from build123d import *

# Parameters (mm, degrees)
F0_W     = 35
F0_H     = 350
F0_R     = 5
F1_DEPTH = 15
F2_W     = 15
F2_H     = 350
F3_DEPTH = 109
F5_DEPTH = 15
F7_DEPTH = 5


with BuildPart() as f1:
    # F0 (on Top) → F1 (new body)
    with BuildSketch(Plane.XY):
        with Locations((-57.72887, 129.090141)):
            Rectangle(F0_W, F0_H)
        with Locations((-50.22887, -15.909859)):
            Circle(F0_R, mode=Mode.SUBTRACT)
        with Locations((-50.22887, 129.090141)):
            Circle(F0_R, mode=Mode.SUBTRACT)
        with Locations((-50.22887, 274.090141)):
            Circle(F0_R, mode=Mode.SUBTRACT)
    extrude(amount=F1_DEPTH)

    # F2 (on face) → F3 (join)
    with BuildSketch(Plane.XY.offset(15)):
        with Locations((-67.72887, 129.090141)):
            Rectangle(F2_W, F2_H)
    extrude(amount=F3_DEPTH)

    # F4 (on face) → F5 (join)
    with BuildSketch(Plane.YZ.offset(-60.22887)):
        Polygon((254.726105, 303.215003), (-45.909859, 124), (304.090141, 124), (304.090141, 332.641874), align=None)
    extrude(amount=-F5_DEPTH)

    # F6 (on face) → F7 (cut)
    with BuildSketch(Plane(origin=(-75.22887, 0, 0), x_dir=(0, -1, 0), z_dir=(-1, 0, 0))):
        Polygon((36.23861, 117.541139), (39.054846, 122.265419), (-304.090141, 326.820885), (-304.090141, 320.417792), align=None)
    extrude(amount=-F7_DEPTH, mode=Mode.SUBTRACT)


solid = f1.part
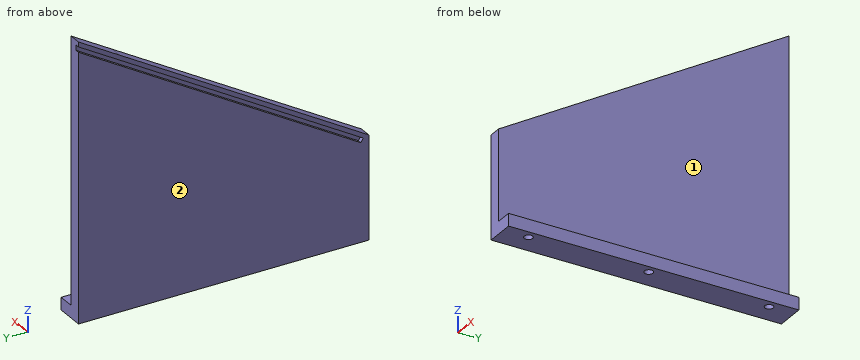
For this review, take the finished solid that the model builds, in its own axes (mm). Face numbers are marked on the shaded views. A direction names the side the tool comes from. Round coordinates to 2 decimals unless told otherwise and drop trailing zeros. Write each loop counter-clockwise with the first axis right and the second up, starting at its lowest first coordinate (ties: lowest second). Pieces come first, ordered by that corner, then holes. Notation, with made-up numbers: (9, 63.5) - (55, 63.5) arc R17 cw to (55, 75.5) - close; hole circle Ø4 at (-15.75, -27). An arc over 180 degrees is marked (long way). Use a Markdown table: item, result.
Q1. Wall thickness on line 1 along Z through (x, y) = (-52, 183.5); line 2 along X through (y, z) = (-18, 119); line 3 along Y through (x, z) = (-72, 221.5): over which ranges is each line inside the solid? List them lowest first.
Derived:
| item | result |
|---|---|
| line 1 | z = 0 to 15 |
| line 2 | x = -75.23 to -60.23 |
| line 3 | y = 117.65 to 127.41, 138.15 to 304.09 |
Q2. Machinability: for the marked faces 1 and 2, which of the approach directions +Z, -Z, +X, -X, +Y, -Y give a long, thin tool a straight path to every point of the face, cutting with its end or side? Answer none if there is none.
Derived:
| item | result |
|---|---|
| face 1 | +Z, +X, +Y, -Y |
| face 2 | +Z, -Z, -X, +Y, -Y |
Q3. Clearance check with flat-ended pins moving along their axes: pin 1 (2 mm diameter, centred on x = -51.5, y = 44.5, fed in from +Z); pin 2 (1 mm diameter, centred on x = -61.5, y = 85, fed in from -Z); pin 3 (2 mm diameter, centred on x = -59.5, y = 182.5, fed in from +Z); pin 4 (8 mm diameter, centred on x = -50.23, y = 274.09, fed in from +Z). State where each tip first meets the part, or that it passes through.
Derived:
| item | result |
|---|---|
| pin 1 | stops at z = 15 |
| pin 2 | stops at z = 0 |
| pin 3 | stops at z = 260.57 |
| pin 4 | passes through |
Q4. We need section B-B (z = 219). Give the boundary of the cut face in (x, y), plus the area to 3 significant figures.
Derived:
| item | result |
|---|---|
| outline | (-75.23, 113.45) - (-60.23, 113.45) - (-60.23, 304.09) - (-75.23, 304.09) - (-75.23, 133.96) - (-70.23, 133.96) - (-70.23, 123.22) - (-75.23, 123.22) - close |
| area | 2,810 mm2 |
Q5. We need section C-C (x = -65.5). Give the boundary of the cut face in (y, z) (3 decimals), plus the area to 3 significant figures.
Derived:
| item | result |
|---|---|
| outline | (-45.91, 0) - (304.09, 0) - (304.09, 332.642) - (-45.91, 124) - close |
| area | 79,900 mm2 |
Q6. We need section D-D (y = 238.5). Give the boundary of the cut face in (x, z), plus the area to 3 significant figures.
Derived:
| item | result |
|---|---|
| outline | (-75.23, 0) - (-40.23, 0) - (-40.23, 15) - (-60.23, 15) - (-60.23, 293.54) - (-75.23, 293.54) - (-75.23, 287.72) - (-70.23, 287.72) - (-70.23, 281.32) - (-75.23, 281.32) - close |
| area | 4,670 mm2 |
Q7. We need section A-A (y = 48.5). Give the boundary of the cut face in (x, z), plus the area to 3 significant figures.
Derived:
| item | result |
|---|---|
| outline | (-75.23, 0) - (-40.23, 0) - (-40.23, 15) - (-60.23, 15) - (-60.23, 180.28) - (-75.23, 180.28) - (-75.23, 174.46) - (-70.23, 174.46) - (-70.23, 168.06) - (-75.23, 168.06) - close |
| area | 2,970 mm2 |
